Geometry check sheet. Reference: the model listing, model coordinates, mm. Face numbers are marked on the shaded views. A direction names the side the tool comes from. Coordinates: 2 decimals unless noted, no trailing zeros. Order: outer loops, then holes, each group sorted by start corner. A loop starts at its lowest first (then second) coordinate and runs counter-clockwise, first axis right, second up. Notation, with made-up numbers: (5, 43) -> (13, 43) arc R16 cw to (13, 69) -> close; hole circle Ø10 at (83.5, 36). An arc over 180 degrees is marked (long way). Answer in a Markdown table with one row per item. Add a question column.
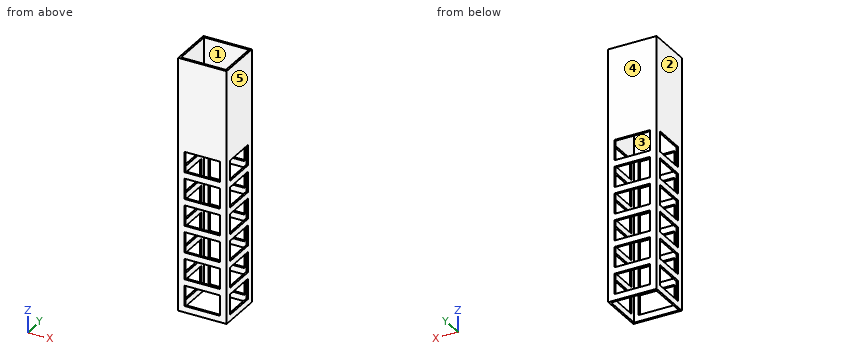
```python
from build123d import *

# Parameters (mm, degrees)
SKETCH1_W           = 190
SKETCH1_H           = 175
SKETCH1_W_2         = 176
SKETCH1_H_2         = 161
BOSS_EXTRUDE1_DEPTH = 496
SKETCH2_W           = 80
SKETCH2_H           = 125
CUT_EXTRUDE1_DEPTH  = 540.487024867
SKETCH5_W           = 140
SKETCH5_H           = 80
CUT_EXTRUDE2_DEPTH  = 535.477314766


with BuildPart() as part:
    # Sketch1 → Boss-Extrude1 (new, symmetric)
    with BuildSketch(Plane.XY):
        with Locations((0, 7)):
            Rectangle(SKETCH1_W, SKETCH1_H)
        with Locations((0, 7)):
            Rectangle(SKETCH1_W_2, SKETCH1_H_2, mode=Mode.SUBTRACT)
    extrude(amount=BOSS_EXTRUDE1_DEPTH, both=True)

    # Sketch2 → Cut-Extrude1 (cut, through all)
    with BuildSketch(Plane(origin=(95, 0, 0), x_dir=(0, 0, -1), z_dir=(1, 0, 0))):
        with Locations((431, 7)):
            Rectangle(SKETCH2_W, SKETCH2_H)
        with Locations((326, 7)):
            Rectangle(SKETCH2_W, SKETCH2_H)
        with Locations((221, 7)):
            Rectangle(SKETCH2_W, SKETCH2_H)
        with Locations((116, 7)):
            Rectangle(SKETCH2_W, SKETCH2_H)
        with Locations((11, 7)):
            Rectangle(SKETCH2_W, SKETCH2_H)
        with Locations((-94, 7)):
            Rectangle(SKETCH2_W, SKETCH2_H)
    extrude(amount=-CUT_EXTRUDE1_DEPTH, mode=Mode.SUBTRACT)

    # Sketch5 → Cut-Extrude2 (cut, through all)
    with BuildSketch(Plane(origin=(0, 94.5, 0), x_dir=(1, 0, 0), z_dir=(0, 1, 0))):
        with Locations((0, 431)):
            Rectangle(SKETCH5_W, SKETCH5_H)
        with Locations((0, 326)):
            Rectangle(SKETCH5_W, SKETCH5_H)
        with Locations((0, 221)):
            Rectangle(SKETCH5_W, SKETCH5_H)
        with Locations((0, 116)):
            Rectangle(SKETCH5_W, SKETCH5_H)
        with Locations((0, 11)):
            Rectangle(SKETCH5_W, SKETCH5_H)
        with Locations((0, -94)):
            Rectangle(SKETCH5_W, SKETCH5_H)
    extrude(amount=-CUT_EXTRUDE2_DEPTH, mode=Mode.SUBTRACT)


solid = part.part
```
(1) Mould release check, pull along Y, two halves, no side actions. Record for the marked faces 3, 4 and 5: +Y half, -Y half, draft (parallel to the pull), parting line (faces both ways), or undercut.
(2) Access from +Z, -Z, +X, -X, +Y, -Y to the whole of each face (thin tool, end or side, straight path). Record for the marked faces 1 and 2.
(3) Cross-section at A-A (z = 396.5). Enter the section's corners in (x, y).
(4) Cross-section at C-C (x = 49). Give the number of separate pieces and of enclosed holes in the cut face, plus the area to 3 significant figures.
(5) Cross-section at B-B (z = -433.5). Enter the section's corners in (x, y).
(6) Scan lines: line 1 along X through (y, z) = (71.5, 397); line 2 along Y through (x, z) = (-26.5, 414.5). Record each from-to range of solid material in increasing order.
Checks:
| question | item | result |
|---|---|---|
| 1 | face 3 | undercut |
| 1 | face 4 | +Y half |
| 1 | face 5 | draft |
| 2 | face 1 | +Z, -Z |
| 2 | face 2 | +Z, -Z, -X, +Y, -Y |
| 3 | outline | (-95, -80.5) -> (95, -80.5) -> (95, 94.5) -> (-95, 94.5) -> close; hole (-88, -73.5) -> (88, -73.5) -> (88, 87.5) -> (-88, 87.5) -> close |
| 4 | separate pieces | 14 |
| 4 | enclosed holes | 0 |
| 4 | area | 7,170 mm² |
| 5 | outline | (-95, -80.5) -> (-70, -80.5) -> (-70, -73.5) -> (-88, -73.5) -> (-88, -55.5) -> (-95, -55.5) -> close; (-95, 69.5) -> (-88, 69.5) -> (-88, 87.5) -> (-70, 87.5) -> (-70, 94.5) -> (-95, 94.5) -> close; (70, -80.5) -> (95, -80.5) -> (95, -55.5) -> (88, -55.5) -> (88, -73.5) -> (70, -73.5) -> close; (70, 87.5) -> (88, 87.5) -> (88, 69.5) -> (95, 69.5) -> (95, 94.5) -> (70, 94.5) -> close |
| 6 | line 1 | -95 to -88, 88 to 95 |
| 6 | line 2 | -80.5 to -73.5, 87.5 to 94.5 |
